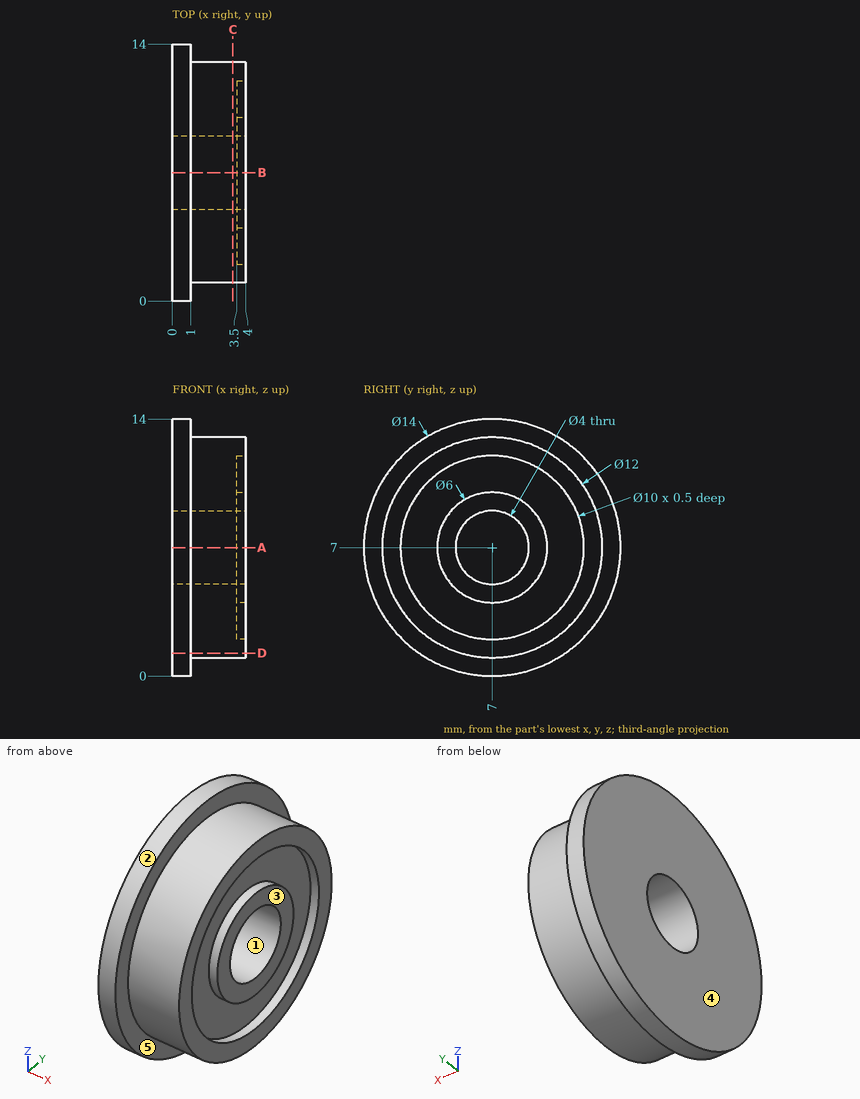
The figure shows three views and two pictorial views of one solid part (mm, origin at its lowest corner). Answer the questions. A direction names the side the tool comes from. Give positions to 0.01 mm unless a question says otherwise; leave off trailing zeros. Loops run counter-clockwise (first coordinate to the right, second up) from the corner with the lowest first, then second, coordinate; pieces in that order, holes last. Notation, with made-up numbers: (74.5, -21) -> (89.5, -21) arc R20 cw to (89.5, 2) -> close; hole circle Ø5 at (24, 31.5). An arc over 180 degrees is marked (long way). Use a Markdown table: item, result. Add a question column.
1. Determine the mould class of the marked faces 1, 2 and 3 for opening direction Y: released by +Y, released by -Y, zero draft, split by the parting line, or undercut.
2. Section C-C on x = 3.3 is taken. Determine the outline of the cut face in (y, z), and give its area (3 significant figures).
3. Flat-ended cylindrical pins translate along their axes: pin 1 Ø1 at (x, z) = (2, 4) entering from +Y; pin 2 Ø1.5 at (x, z) = (2.5, 8.5) entering from +Y. Find the tip coordinate at first contact, or state that the pin passes through.
4. Section A-A on z = 7 is taken. Determine the outline of the cut face in (x, y), and give its area (3 significant figures).
5. Section D-D on z = 1.25 is taken. Determine the outline of the cut face in (x, y), and give its area (3 significant figures).
6. For the marked faces 4 and 5, determine the directions among +Z, -Z, +X, -X, +Y, -Y from which every point of the face is accessible in a straight line to the end or side of a thin tool.
7. Find the intervals of material crossed by probe 1 along Y at (x, z) = (3.8, 7); probe 2 along X at (y, z) = (8.75, 13.25); probe 3 along Y at (x, z) = (3.85, 8.75), in increasing order.
Results below:
| question | item | result |
|---|---|---|
| 1 | face 1 | undercut |
| 1 | face 2 | split by the parting line |
| 1 | face 3 | zero draft |
| 2 | outline | circle Ø12 at (7, 7); hole circle Ø4 at (7, 7) |
| 2 | area | 101 mm^2 |
| 3 | pin 1 | stops at y = 12.45 |
| 3 | pin 2 | stops at y = 12.95 |
| 4 | outline | (0, 0) -> (1, 0) -> (1, 1) -> (4, 1) -> (4, 2) -> (3.5, 2) -> (3.5, 4) -> (4, 4) -> (4, 5) -> (0, 5) -> close; (0, 9) -> (4, 9) -> (4, 10) -> (3.5, 10) -> (3.5, 12) -> (4, 12) -> (4, 13) -> (1, 13) -> (1, 14) -> (0, 14) -> close |
| 4 | area | 32.0 mm^2 |
| 5 | outline | (0, 3.01) -> (1, 3.01) -> (1, 5.29) -> (4, 5.29) -> (4, 8.71) -> (1, 8.71) -> (1, 10.99) -> (0, 10.99) -> close |
| 5 | area | 18.3 mm^2 |
| 6 | face 4 | +Z, -Z, -X, +Y, -Y |
| 6 | face 5 | +X |
| 7 | probe 1 | y = 1 to 2, 4 to 5, 9 to 10, 12 to 13 |
| 7 | probe 2 | x = 0 to 1 |
| 7 | probe 3 | y = 1.26 to 2.32, 4.56 to 6.03, 7.97 to 9.44, 11.68 to 12.74 |
